Check sheet for the modelled part. Datum: model origin and axes. Units: mm. A direction names the side the tool comes from. Coordinates: 2 decimals unless noted, no trailing zeros. Loops run counter-clockwise (first coordinate to the right, second up) from the corner with the lowest first, then second, coordinate; pieces in that order, holes last. Notation, with made-up numbers: (-4, -19.75) -> (14, -19.75) arc R15 ccw to (14, -12.75) -> close; hole circle Ø9 at (3, -8). An arc over 180 degrees is marked (long way). Use CSV: the item, a comma, the result in double quotes. Start each with the question number.
1. Sectioned sample at C-C, the plane y = 66.5. Record the cut outline in (x, z).
2. Release check for a two-part mould opening along Y. For faces 1 (the face through (0, 89, 0)), 2 (the face through (0, -1, 0)), 3 (the face through (-2, 0, -1.3)) record: pulls with the +Y half, pulls with the -Y half, needs draft (parallel to the pull), parting line crosses it, or undercut.
3. Thickness scan on L1, parallel to Z at x = -0.05, y = 37.5; L2, parallel to X at y = 88, z = 0.35. Record the ranges inside material, lowest first.
4. Gauge pin test, flat end, axial feed: pin 1 (1 mm diameter, centred on y = 10, z = 1.5, fed in from -X). Record the tip position at first contact, or that the pin passes through.
5. Sectioned sample at D-D, the plane y = 88. Record the cut outline in (x, z).
6. Sectioned sample at B-B, the plane x = 0. Record the cut outline in (y, z).
7. Set-up check for faces 4 (the face through (1.308, 44.124, 1.706)), 5 (the face through (0, 90, 0)): record each of +Z, -Z, +X, -X, +Y, -Y from which the full face is reachable in a straight line by a thin tool's end or side.
8. Sectioned sample at A-A, the plane z = 0. Record the cut outline in (x, y), and give its area (3 significant figures).
```python
from build123d import *

# Parameters (mm, degrees)
SKETCH1_R               = 2.15
BOSS_EXTRUDE1_DEPTH     = 90
CHAMFER1_SIZE           = 0.5
SKETCH2_R               = 3
BOSS_EXTRUDE2_DEPTH     = 1
CUT_EXTRUDE1_DEPTH      = 91.099944506
CUT_EXTRUDE1_DEPTH_BACK = 91.099944506
SKETCH3_R               = 1


with BuildPart() as part:
    # Sketch1 → Boss-Extrude1 (new body)
    with BuildSketch(Plane(origin=(0, 0, 0), x_dir=(1, 0, 0), z_dir=(0, 1, 0))):
        with Locations(Location((0, 0, 0), (0, 0, 90))):
            Circle(SKETCH1_R)
    extrude(amount=BOSS_EXTRUDE1_DEPTH)

    # Chamfer1
    chamfer1_edges = [part.edges().sort_by_distance(p)[0] for p in [
        (0, 90, 2.15),
    ]]
    chamfer(chamfer1_edges, length=CHAMFER1_SIZE)

    # Sketch2 → Boss-Extrude2 (add)
    with BuildSketch(Plane(origin=(0, 0, 0), x_dir=(-1, 0, 0), z_dir=(0, -1, 0))):
        with Locations(Location((0, 0, 0), (0, 0, 90))):
            Circle(SKETCH2_R)
    extrude(amount=BOSS_EXTRUDE2_DEPTH)

    # Sketch3 → Cut-Extrude1 (cut, two sides: drawn at the far end of the back side and taken through both)
    with BuildSketch(Plane.XY.offset(-CUT_EXTRUDE1_DEPTH_BACK)):
        with Locations(Location((0, 88, 0), (0, 0, 89.999999996))):
            Circle(SKETCH3_R)
    extrude(amount=CUT_EXTRUDE1_DEPTH + CUT_EXTRUDE1_DEPTH_BACK, mode=Mode.SUBTRACT)


solid = part.part
```
Completed:
1,outline,"circle Ø4.3 at (0, 0)"
2,face 1,"undercut"
2,face 2,"pulls with the -Y half"
2,face 3,"pulls with the +Y half"
3,L1,"-2.15 to 2.15"
3,L2,"-2.12 to -1, 1 to 2.12"
4,pin 1,"x = -1.9"
5,outline,"(-1, -1.9) -> (-1, 1.9) arc R2.15 ccw to start; (1, -1.9) arc R2.15 ccw to (1, 1.9) -> close"
6,outline,"(-1, -3) -> (0, -3) -> (0, -2.15) -> (87, -2.15) -> (87, 2.15) -> (0, 2.15) -> (0, 3) -> (-1, 3) -> close; (89, -2.15) -> (89.5, -2.15) -> (90, -1.65) -> (90, 1.65) -> (89.5, 2.15) -> (89, 2.15) -> close"
7,face 4,"+Y"
7,face 5,"+Z, -Z, +X, -X, +Y"
8,outline,"(-3, -1) -> (3, -1) -> (3, 0) -> (2.15, 0) -> (2.15, 89.5) -> (1.65, 90) -> (-1.65, 90) -> (-2.15, 89.5) -> (-2.15, 0) -> (-3, 0) -> close; hole circle Ø2 at (0, 88)"
8,area,"390 mm²"
